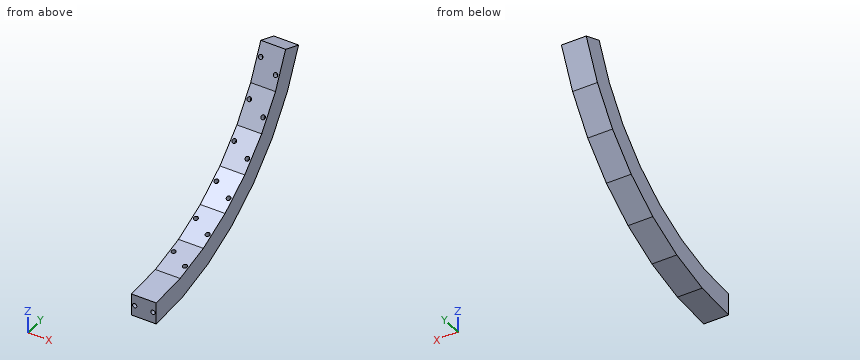
Autodesk Inventor part; units mm, degrees
ref_plane "YZ Plane" through (0, 0, 0) normal (1, 0, 0) x (0, 1, 0)
ref_plane "XZ Plane" through (0, 0, 0) normal (0, 1, 0) x (-1, 0, 0)
ref_plane "XY Plane" through (0, 0, 0) normal (0, 0, 1) x (1, 0, 0)
sketch "Sketch1" plane through (0, 0, 0) normal (1, 0, 0) x (0, 1, 0)
  circle A0 centre (0, 0) radius 200 construction
  line L0 (0, 0) -> (293, 0) construction
  line L1 (0, 0) -> (315, -114.6506) construction
  line L2 (0, 0) -> (335.216, 0) construction
  line L3 (0, -200) -> (-34.7296, -196.9616)
  line L4 (-34.7296, -196.9616) -> (-68.404, -187.9385)
  line L5 (-68.404, -187.9385) -> (-100, -173.2051)
  line L6 (-100, -173.2051) -> (-128.5575, -153.2089)
  line L7 (-128.5575, -153.2089) -> (-153.2089, -128.5575)
  line L8 (-153.2089, -128.5575) -> (-173.2051, -100)
  line L9 (-173.2051, -100) -> (-187.9385, -68.404)
  line L10 (-187.9385, -68.404) -> (-196.9616, -34.7296)
  line L11 (-196.9616, -34.7296) -> (-200, 0)
  line L12 (-200, 0) -> (-196.9616, 34.7296)
  line L13 (-196.9616, 34.7296) -> (-187.9385, 68.404)
  line L14 (-187.9385, 68.404) -> (-173.2051, 100)
  line L15 (-173.2051, 100) -> (-153.2089, 128.5575)
  line L16 (-153.2089, 128.5575) -> (-128.5575, 153.2089)
  line L17 (-128.5575, 153.2089) -> (-100, 173.2051)
  line L18 (-100, 173.2051) -> (-68.404, 187.9385)
  line L19 (-68.404, 187.9385) -> (-34.7296, 196.9616)
  line L20 (-34.7296, 196.9616) -> (0, 200)
  line L21 (0, 200) -> (34.7296, 196.9616)
  line L22 (34.7296, 196.9616) -> (68.404, 187.9385)
  line L23 (68.404, 187.9385) -> (100, 173.2051)
  line L24 (100, 173.2051) -> (128.5575, 153.2089)
  line L25 (128.5575, 153.2089) -> (153.2089, 128.5575)
  line L26 (153.2089, 128.5575) -> (173.2051, 100)
  line L27 (173.2051, 100) -> (187.9385, 68.404)
  line L28 (187.9385, 68.404) -> (196.9616, 34.7296)
  line L29 (196.9616, 34.7296) -> (200, 0)
  line L30 (200, 0) -> (196.9616, -34.7296)
  line L31 (196.9616, -34.7296) -> (187.9385, -68.404)
  line L32 (187.9385, -68.404) -> (173.2051, -100)
  line L33 (173.2051, -100) -> (153.2089, -128.5575)
  line L34 (153.2089, -128.5575) -> (128.5575, -153.2089)
  line L35 (128.5575, -153.2089) -> (100, -173.2051)
  line L36 (100, -173.2051) -> (68.404, -187.9385)
  line L37 (68.404, -187.9385) -> (34.7296, -196.9616)
  line L38 (34.7296, -196.9616) -> (0, -200)
  circle A1 centre (0, 0) radius 220 construction
  line L39 (0, -220) -> (-38.2026, -216.6577)
  line L40 (-38.2026, -216.6577) -> (-75.2444, -206.7324)
  line L41 (-75.2444, -206.7324) -> (-110, -190.5256)
  line L42 (-110, -190.5256) -> (-141.4133, -168.5298)
  line L43 (-141.4133, -168.5298) -> (-168.5298, -141.4133)
  line L44 (-168.5298, -141.4133) -> (-190.5256, -110)
  line L45 (-190.5256, -110) -> (-206.7324, -75.2444)
  line L46 (-206.7324, -75.2444) -> (-216.6577, -38.2026)
  line L47 (-216.6577, -38.2026) -> (-220, 0)
  line L48 (-220, 0) -> (-216.6577, 38.2026)
  line L49 (-216.6577, 38.2026) -> (-206.7324, 75.2444)
  line L50 (-206.7324, 75.2444) -> (-190.5256, 110)
  line L51 (-190.5256, 110) -> (-168.5298, 141.4133)
  line L52 (-168.5298, 141.4133) -> (-141.4133, 168.5298)
  line L53 (-141.4133, 168.5298) -> (-110, 190.5256)
  line L54 (-110, 190.5256) -> (-75.2444, 206.7324)
  line L55 (-75.2444, 206.7324) -> (-38.2026, 216.6577)
  line L56 (-38.2026, 216.6577) -> (0, 220)
  line L57 (0, 220) -> (38.2026, 216.6577)
  line L58 (38.2026, 216.6577) -> (75.2444, 206.7324)
  line L59 (75.2444, 206.7324) -> (110, 190.5256)
  line L60 (110, 190.5256) -> (141.4133, 168.5298)
  line L61 (141.4133, 168.5298) -> (168.5298, 141.4133)
  line L62 (168.5298, 141.4133) -> (190.5256, 110)
  line L63 (190.5256, 110) -> (206.7324, 75.2444)
  line L64 (206.7324, 75.2444) -> (216.6577, 38.2026)
  line L65 (216.6577, 38.2026) -> (220, 0)
  line L66 (220, 0) -> (216.6577, -38.2026)
  line L67 (216.6577, -38.2026) -> (206.7324, -75.2444)
  line L68 (206.7324, -75.2444) -> (190.5256, -110)
  line L69 (190.5256, -110) -> (168.5298, -141.4133)
  line L70 (168.5298, -141.4133) -> (141.4133, -168.5298)
  line L71 (141.4133, -168.5298) -> (110, -190.5256)
  line L72 (110, -190.5256) -> (75.2444, -206.7324)
  line L73 (75.2444, -206.7324) -> (38.2026, -216.6577)
  line L74 (38.2026, -216.6577) -> (0, -220)
  line L75 (0, -200) -> (0, -220)
  line L76 (187.9385, -68.404) -> (206.7324, -75.2444)
  dimension "d0" = 400
  dimension "d2" = 440
  dimension "d1" = 20
extrude "Extrusion1" add sketch "Sketch1" against normal blind 23 contours L38 L37 L36 L35 L34 L33 L32 L76 L68 L69 L70 L71 L72 L73 L74 L75
sketch "Sketch2" plane through (-23, 34.7296, -196.9616) normal (0, -0.0871557, 0.9961947) x (1, 0, 0)
  line L0 (23, 0) -> (23, -34.8623)
  line L1 (23, 0) -> (0, 0)
  line L2 (0, -34.8623) -> (0, 0)
  line L3 (23, -34.8623) -> (0, -34.8623)
  line L4 (0, -33.9311) -> (23, -33.9311)
  line L5 (23, -33.9311) -> (23, -0.9311)
  line L6 (23, -0.9311) -> (0, -0.9311)
  line L7 (0, -0.9311) -> (0, -33.9311)
  line L8 (0, -33.9311) -> (23, -0.9311) construction
  line L9 (23, -33.9311) -> (0, -0.9311) construction
  point P0 (23, -17.4311)
  point P1 (11.5, -17.4311)
  point P2 (3.4356, -12.6296)
  point P3 (19.8273, -22.2197)
  dimension "d5" = 34.8623
  dimension "d6" = 23
  dimension "d7" = 23
  dimension "d8" = 33
  dimension "d10" = 3.4356
  dimension "d11" = 21.3015
  dimension "d12" = 19.8273
  dimension "d13" = 11.7114
sketch "Sketch9" plane through (-23.1315, 68.3978, -187.9402) normal (0, -0.258819, 0.9659258) x (1, 0, 0)
  line L0 (23, 0) -> (23, -34.8623)
  line L1 (23, 0) -> (0, 0)
  line L2 (0, -34.8623) -> (0, 0)
  line L3 (23, -34.8623) -> (0, -34.8623)
  line L4 (0, -33.9311) -> (23, -33.9311)
  line L5 (23, -33.9311) -> (23, -0.9311)
  line L6 (23, -0.9311) -> (0, -0.9311)
  line L7 (0, -0.9311) -> (0, -33.9311)
  line L8 (0, -33.9311) -> (23, -0.9311) construction
  line L9 (23, -33.9311) -> (0, -0.9311) construction
  point P0 (23, -17.4311)
  point P1 (11.5, -17.4311)
  point P2 (3.4356, -12.6296)
  point P3 (19.8273, -22.2197)
  dimension "d124" = 34.8623
  dimension "d125" = 23
  dimension "d116" = 23
  dimension "d117" = 33
  dimension "d115" = 3.4356
  dimension "d114" = 21.3015
  dimension "d113" = 19.8273
  dimension "d112" = 11.7114
hole "Hole8" at (-19.6959, 56.1985, -191.209) at (-3.3042, 46.9352, -193.6911) direction (0, 0.258819, -0.9659258) diameter 4 depth 6
sketch "Sketch10" plane through (-23.1315, 99.9942, -173.2078) normal (0, -0.4226183, 0.9063078) x (1, 0, 0)
  line L0 (23, 0) -> (23, -34.8623)
  line L1 (23, 0) -> (0, 0)
  line L2 (0, -34.8623) -> (0, 0)
  line L3 (23, -34.8623) -> (0, -34.8623)
  line L4 (0, -33.9311) -> (23, -33.9311)
  line L5 (23, -33.9311) -> (23, -0.9311)
  line L6 (23, -0.9311) -> (0, -0.9311)
  line L7 (0, -0.9311) -> (0, -33.9311)
  line L8 (0, -33.9311) -> (23, -0.9311) construction
  line L9 (23, -33.9311) -> (0, -0.9311) construction
  point P0 (23, -17.4311)
  point P1 (11.5, -17.4311)
  point P2 (3.4356, -12.6296)
  point P3 (19.8273, -22.2197)
  dimension "d139" = 34.8623
  dimension "d140" = 23
  dimension "d131" = 23
  dimension "d132" = 33
  dimension "d130" = 3.4356
  dimension "d129" = 21.3015
  dimension "d128" = 19.8273
  dimension "d127" = 11.7114
hole "Hole9" at (-19.6959, 88.5478, -178.5453) at (-3.3042, 79.8562, -182.5983) direction (0, 0.4226183, -0.9063078) diameter 4 depth 6
sketch "Sketch11" plane through (-23.1315, 128.5522, -153.2126) normal (0, -0.5735764, 0.819152) x (1, 0, 0)
  line L0 (23, 0) -> (23, -34.8623)
  line L1 (23, 0) -> (0, 0)
  line L2 (0, -34.8623) -> (0, 0)
  line L3 (23, -34.8623) -> (0, -34.8623)
  line L4 (0, -33.9311) -> (23, -33.9311)
  line L5 (23, -33.9311) -> (23, -0.9311)
  line L6 (23, -0.9311) -> (0, -0.9311)
  line L7 (0, -0.9311) -> (0, -33.9311)
  line L8 (0, -33.9311) -> (23, -0.9311) construction
  line L9 (23, -33.9311) -> (0, -0.9311) construction
  point P0 (23, -17.4311)
  point P1 (11.5, -17.4311)
  point P2 (3.4356, -12.6296)
  point P3 (19.8273, -22.2197)
  dimension "d154" = 34.8623
  dimension "d155" = 23
  dimension "d146" = 23
  dimension "d147" = 33
  dimension "d145" = 3.4356
  dimension "d144" = 21.3015
  dimension "d143" = 19.8273
  dimension "d142" = 11.7114
hole "Hole10" at (-19.6959, 118.2066, -160.4567) at (-3.3042, 110.3509, -165.9573) direction (0, 0.5735764, -0.819152) diameter 4 depth 6
sketch "Sketch12" plane through (-23.1315, 153.2043, -128.5621) normal (0, -0.7071068, 0.7071068) x (1, 0, 0)
  line L0 (23, 0) -> (23, -34.8623)
  line L1 (23, 0) -> (0, 0)
  line L2 (0, -34.8623) -> (0, 0)
  line L3 (23, -34.8623) -> (0, -34.8623)
  line L4 (0, -33.9311) -> (23, -33.9311)
  line L5 (23, -33.9311) -> (23, -0.9311)
  line L6 (23, -0.9311) -> (0, -0.9311)
  line L7 (0, -0.9311) -> (0, -33.9311)
  line L8 (0, -33.9311) -> (23, -0.9311) construction
  line L9 (23, -33.9311) -> (0, -0.9311) construction
  point P0 (23, -17.4311)
  point P1 (11.5, -17.4311)
  point P2 (3.4356, -12.6296)
  point P3 (19.8273, -22.2197)
  dimension "d169" = 34.8623
  dimension "d170" = 23
  dimension "d161" = 23
  dimension "d162" = 33
  dimension "d160" = 3.4356
  dimension "d159" = 21.3015
  dimension "d158" = 19.8273
  dimension "d157" = 11.7114
hole "Hole11" at (-19.6959, 144.2738, -137.4926) at (-3.3042, 137.4926, -144.2738) direction (0, 0.7071068, -0.7071068) diameter 4 depth 6
sketch "Sketch13" plane through (-23.1315, 173.2014, -100.0053) normal (0, -0.819152, 0.5735764) x (1, 0, 0)
  line L0 (23, 0) -> (23, -34.8623)
  line L1 (23, 0) -> (0, 0)
  line L2 (0, -34.8623) -> (0, 0)
  line L3 (23, -34.8623) -> (0, -34.8623)
  line L4 (0, -33.9311) -> (23, -33.9311)
  line L5 (23, -33.9311) -> (23, -0.9311)
  line L6 (23, -0.9311) -> (0, -0.9311)
  line L7 (0, -0.9311) -> (0, -33.9311)
  line L8 (0, -33.9311) -> (23, -0.9311) construction
  line L9 (23, -33.9311) -> (0, -0.9311) construction
  point P0 (23, -17.4311)
  point P1 (11.5, -17.4311)
  point P2 (3.4356, -12.6296)
  point P3 (19.8273, -22.2197)
  dimension "d184" = 34.8623
  dimension "d185" = 23
  dimension "d176" = 23
  dimension "d177" = 33
  dimension "d175" = 3.4356
  dimension "d174" = 21.3015
  dimension "d173" = 19.8273
  dimension "d172" = 11.7114
hole "Hole12" at (-19.6959, 165.9573, -110.3509) at (-3.3042, 160.4567, -118.2066) direction (0, 0.819152, -0.5735764) diameter 4 depth 6
sketch "Sketch14" plane through (-23.1315, 187.9358, -68.4099) normal (0, -0.9063078, 0.4226183) x (1, 0, 0)
  line L0 (23, 0) -> (23, -34.8623)
  line L1 (23, 0) -> (0, 0)
  line L2 (0, -34.8623) -> (0, 0)
  line L3 (23, -34.8623) -> (0, -34.8623)
  line L4 (0, -33.9311) -> (23, -33.9311)
  line L5 (23, -33.9311) -> (23, -0.9311)
  line L6 (23, -0.9311) -> (0, -0.9311)
  line L7 (0, -0.9311) -> (0, -33.9311)
  line L8 (0, -33.9311) -> (23, -0.9311) construction
  line L9 (23, -33.9311) -> (0, -0.9311) construction
  point P0 (23, -17.4311)
  point P1 (11.5, -17.4311)
  point P2 (3.4356, -12.6296)
  point P3 (19.8273, -22.2197)
  dimension "d199" = 34.8623
  dimension "d200" = 23
  dimension "d191" = 23
  dimension "d192" = 33
  dimension "d190" = 3.4356
  dimension "d189" = 21.3015
  dimension "d188" = 19.8273
  dimension "d187" = 11.7114
hole "Hole13" at (-19.6959, 182.5983, -79.8562) at (-3.3042, 178.5453, -88.5478) direction (0, 0.9063078, -0.4226183) diameter 4 depth 6
sketch "Sketch15" plane through (0, 0, -220) normal (0, -1, 0) x (1, 0, 0)
  line L0 (0, 20) -> (0, 0)
  line L1 (0, 20) -> (-23, 20)
  line L2 (-23, 0) -> (-23, 20)
  line L3 (0, 0) -> (-23, 0)
  point P0 (0, 220)
  point P1 (-3, 10)
  point P2 (-20, 10)
  dimension "d201" = 3
  dimension "d202" = 3
hole "Hole14" at (-20, 0, -210) at (-3, 0, -210) direction (0, 1, 0) diameter 4 depth 6 tip angle 118
equation "\"d116\" = d7"
equation "\"d117\" = d8"
equation "\"d123\" = d14"
equation "\"d122\" = d19"
equation "\"d131\" = d7"
equation "\"d132\" = d8"
equation "\"d138\" = d14"
equation "\"d137\" = d19"
equation "\"d146\" = d7"
equation "\"d147\" = d8"
equation "\"d153\" = d14"
equation "\"d152\" = d19"
equation "\"d161\" = d7"
equation "\"d162\" = d8"
equation "\"d168\" = d14"
equation "\"d167\" = d19"
equation "\"d176\" = d7"
equation "\"d177\" = d8"
equation "\"d183\" = d14"
equation "\"d182\" = d19"
equation "\"d191\" = d7"
equation "\"d192\" = d8"
equation "\"d198\" = d14"
equation "\"d197\" = d19"
properties part number "fourche_v2_sans_radiateurs"
Could you check a few things on this model? Use its own coordinates, in mm. Give positions to 0.01 mm unless a question says otherwise; leave off trailing zeros. Loops run counter-clockwise (first coordinate to the right, second up) from the corner with the lowest first, then second, coordinate; pieces in that order, holes last. Notation, with made-up numbers: (-34.75, 38) - (11.25, 38) arc R26 ccw to (11.25, 71) - close; hole circle Ø6 at (20, -40). An arc over 180 degrees is marked (long way). Use one line per item in the form item = value.
1. I'm going to push flat-ended pins straight in: pin 1 Ø1.5 at (x, y) = (-12.5, 81.5) entering from +Z; pin 2 Ø8 at (x, z) = (-10.5, -150.5) entering from -Y; pin 3 Ø8 at (x, z) = (-11, -165.5) entering from +Y. Where does each tip first touch, or does it pass through?
Response values:
pin_1 = -181.48
pin_2 = 126.71
pin_3 = 148.44
2. I need wall thicknesses on probe 1 along X at (y, z) = (3, -210); probe 2 along Z at (x, y) = (-3, 2.1); probe 3 along Y at (x, z) = (-21.25, -183.5). Which ranges of each line are inside material? Lowest first, please.
Response values:
probe_1 = -23 to -22, -18 to -5, -1 to 0
probe_2 = -219.82 to -212, -208 to -199.82
probe_3 = 77.92 to 89.47, 92.12 to 120.03
3. I want a section at A-A (z = -96). Please give me the cut outline in (x, y), and give its area (3 significant figures).
Response values:
outline = (-23, 175.07) - (0, 175.07) - (0, 197.05) - (-23, 197.05) - close
area = 506 mm²
